from build123d import *

# Parameters (mm, degrees)
SKETCH1_R                   = 18.542
EXTRUDE1_DEPTH              = 19.05
SKETCH2_R                   = 13.335
CUT_EXTRUDE1_DEPTH          = 13.86078
CUT_EXTRUDE1_DRAFT          = -1.783333333
SKETCH5_R                   = 14.242142857
CUT_EXTRUDE3_DEPTH          = 3.175
CUT_EXTRUDE3_DRAFT          = -45
CIRPATTERN1_COPY_1_SKETCH_R = 13.335
CIRPATTERN1_COPY_1_DEPTH    = 13.86078
CIRPATTERN1_COPY_1_DRAFT    = -1.783333333
CIRPATTERN1_COPY_2_SKETCH_R = 14.242142857
CIRPATTERN1_COPY_2_DEPTH    = 3.175
CIRPATTERN1_COPY_2_DRAFT    = -45
FILLET1_R                   = 0.381
SKETCH8_R                   = 12.903443323
CUT_EXTRUDE5_DEPTH          = 36.709260955


with BuildPart() as part:
    # Sketch1 → Extrude1 (new, symmetric)
    with BuildSketch(Plane.XY):
        with Locations(Location((0, 0, 0), (0, 0, 180))):
            Circle(SKETCH1_R)
    extrude(amount=EXTRUDE1_DEPTH, both=True)


with BuildPart() as cut_extrude1_tool:
    # Sketch2 → Cut-Extrude1 (with draft: the straight prism first)
    with BuildSketch(Plane.XY.offset(19.05)):
        Circle(SKETCH2_R)
    extrude(amount=-CUT_EXTRUDE1_DEPTH)
    # Cut-Extrude1: the draft: its side faces are tilted about the plane it starts from
    cut_extrude1_sides = [cut_extrude1_tool.faces().sort_by_distance(p)[0] for p in [
        (-13.335, 0, 12.11961),
    ]]
    draft(cut_extrude1_sides, Plane.XY.offset(19.05), CUT_EXTRUDE1_DRAFT)


with BuildPart() as part_1:
    add(part.part)

    # Cut-Extrude1: cut by cut_extrude1_tool
    add(cut_extrude1_tool.part, mode=Mode.SUBTRACT)


with BuildPart() as cut_extrude3_tool:
    # Sketch5 → Cut-Extrude3 (with draft: the straight prism first)
    with BuildSketch(Plane.XY.offset(19.05)):
        Circle(SKETCH5_R)
    extrude(amount=-CUT_EXTRUDE3_DEPTH)
    # Cut-Extrude3: the draft: its side faces are tilted about the plane it starts from
    cut_extrude3_sides = [cut_extrude3_tool.faces().sort_by_distance(p)[0] for p in [
        (-14.242142857, 0, 17.4625),
    ]]
    draft(cut_extrude3_sides, Plane.XY.offset(19.05), CUT_EXTRUDE3_DRAFT)


with BuildPart() as part_2:
    add(part_1.part)

    # Cut-Extrude3: cut by cut_extrude3_tool
    add(cut_extrude3_tool.part, mode=Mode.SUBTRACT)


with BuildPart() as cirpattern1_copy_1_tool:
    # CirPattern1 copy 1 sketch → CirPattern1 copy 1 (with draft: the straight prism first)
    with BuildSketch(Plane(origin=(0, 0, -19.05), x_dir=(-1, 0, 0), z_dir=(0, 0, -1))):
        Circle(CIRPATTERN1_COPY_1_SKETCH_R)
    extrude(amount=-CIRPATTERN1_COPY_1_DEPTH)
    # CirPattern1 copy 1: the draft: its side faces are tilted about the plane it starts from
    cirpattern1_copy_1_sides = [cirpattern1_copy_1_tool.faces().sort_by_distance(p)[0] for p in [
        (13.335, 0, -12.11961),
    ]]
    draft(cirpattern1_copy_1_sides, Plane(origin=(0, 0, -19.05), x_dir=(-1, 0, 0), z_dir=(0, 0, -1)), CIRPATTERN1_COPY_1_DRAFT)


with BuildPart() as part_3:
    add(part_2.part)

    # CirPattern1 copy 1: cut by cirpattern1_copy_1_tool
    add(cirpattern1_copy_1_tool.part, mode=Mode.SUBTRACT)


with BuildPart() as cirpattern1_copy_2_tool:
    # CirPattern1 copy 2 sketch → CirPattern1 copy 2 (with draft: the straight prism first)
    with BuildSketch(Plane(origin=(0, 0, -19.05), x_dir=(-1, 0, 0), z_dir=(0, 0, -1))):
        Circle(CIRPATTERN1_COPY_2_SKETCH_R)
    extrude(amount=-CIRPATTERN1_COPY_2_DEPTH)
    # CirPattern1 copy 2: the draft: its side faces are tilted about the plane it starts from
    cirpattern1_copy_2_sides = [cirpattern1_copy_2_tool.faces().sort_by_distance(p)[0] for p in [
        (14.242142857, 0, -17.4625),
    ]]
    draft(cirpattern1_copy_2_sides, Plane(origin=(0, 0, -19.05), x_dir=(-1, 0, 0), z_dir=(0, 0, -1)), CIRPATTERN1_COPY_2_DRAFT)


with BuildPart() as part_4:
    add(part_3.part)

    # CirPattern1 copy 2: cut by cirpattern1_copy_2_tool
    add(cirpattern1_copy_2_tool.part, mode=Mode.SUBTRACT)

    # Fillet1
    fillet1_edges = [part_4.edges().sort_by_distance(p)[0] for p in [
        (18.542, 0, -19.05),
        (18.542, 0, 19.05),
    ]]
    fillet(fillet1_edges, radius=FILLET1_R)

    # Sketch8 → Cut-Extrude5 (cut, through all)
    with BuildSketch(Plane.XY.offset(5.18922)):
        Circle(SKETCH8_R)
    extrude(amount=-CUT_EXTRUDE5_DEPTH, mode=Mode.SUBTRACT)


solid = part_4.part
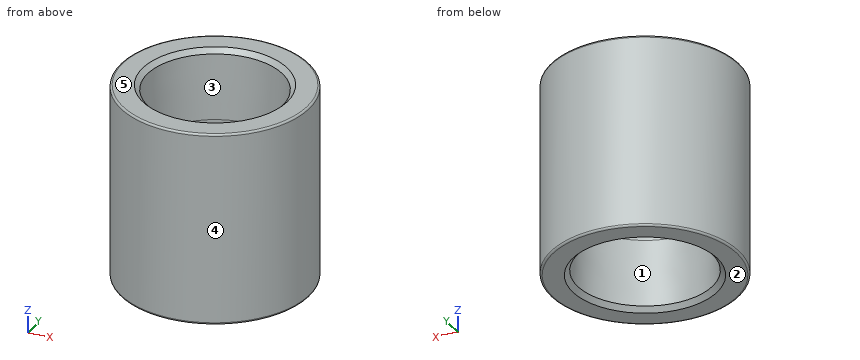
CAD build for the part. Positions are in the model's coordinates, mm. Face numbers are marked on the shaded views. A direction names the side the tool comes from. Round coordinates to 2 decimals unless told otherwise and drop trailing zeros. Loops run counter-clockwise (first coordinate to the right, second up) from the corner with the lowest first, then second, coordinate; pieces in that order, holes last.
(1) Drop flat-ended pins along their axis: pin 1 (12 mm diameter, centred on x = -11, y = -8, fed in from +Z); pin 2 (20.5 mm diameter, centred on x = 0, y = 0, fed in from -Z); pin 3 (2 mm diameter, centred on y = 2.5, z = 8.5, fed in from -X); pin 4 (12 mm diameter, centred on x = 9.5, z = -0.5, fed in from +Y). Give the stop position or say it passes through.
(2) Wall check: line 1 along Y through (x, z) = (0, 0.5); line 2 along X through (y, z) = (2.5, 17); line 3 along Y through (x, z) = (4, -8.5). Give the ranges that are in metal, low to high.
(3) Which spindle directions (+Z, -Z, +X, -X, +Y, -Y) get a long thin tool onto all of the face, cutting with end or side? Do the marked faces 1 and 2. Say none if no direction does.
(4) Cut at C-C (z = -2.5). Give the cut face in (x, y).
(5) Cut at A-A (x = 0). Give the cut face in (y, z).
(6) Two-plate mould, pull along Y, no slides. Class the marked faces 3, 4 and 5: +Y half, -Y half, draft (parallel to the pull), parting line (faces both ways), or undercut.
(7) Cut at D-D (z = 10). Give the cut face in (x, y), plus the area to 3 significant figures.
Findings below:
1. pin 1: stops at z = 19.05
1. pin 2: passes through
1. pin 3: stops at x = -18.48
1. pin 4: stops at y = 18.21
2. line 1: y = -18.54 to -12.9, 12.9 to 18.54
2. line 2: x = -18.37 to -13.03, 13.03 to 18.37
2. line 3: y = -18.11 to -12.38, 12.38 to 18.11
3. face 1: -Z
3. face 2: -Z, +X, -X, +Y, -Y
4. outline: circle Ø37.08 at (0, 0); hole circle Ø25.81 at (0, 0)
5. outline: (-18.54, -18.67) arc R0.38 ccw to (-18.16, -19.05) - (-14.24, -19.05) - (-13.31, -18.11) - (-12.9, -5.19) - (-12.9, 5.19) - (-13.31, 18.11) - (-14.24, 19.05) - (-18.16, 19.05) arc R0.38 ccw to (-18.54, 18.67) - close; (12.9, -5.19) - (13.31, -18.11) - (14.24, -19.05) - (18.16, -19.05) arc R0.38 ccw to (18.54, -18.67) - (18.54, 18.67) arc R0.38 ccw to (18.16, 19.05) - (14.24, 19.05) - (13.31, 18.11) - (12.9, 5.19) - close
6. face 3: undercut
6. face 4: parting line
6. face 5: draft
7. outline: circle Ø37.08 at (0, 0); hole circle Ø26.11 at (0, 0)
7. area: 545 mm2
